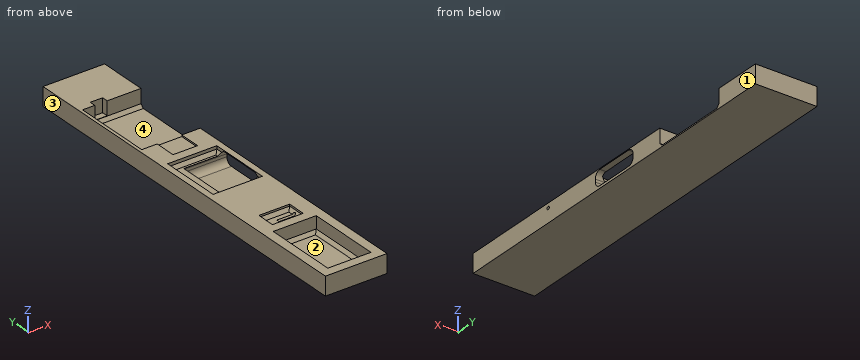
```python
from build123d import *

# Parameters (mm, degrees)
BOX038_W          = 4
BOX038_H          = 4
BOX038_DEPTH      = 10
BOX037_W          = 3
BOX037_H          = 6
BOX037_DEPTH      = 10
BOX036_W          = 2
BOX036_H          = 2.5
BOX036_DEPTH      = 10
BOX027_W          = 8.65
BOX027_H          = 8.3
BOX027_DEPTH      = 2.45
FILLET016_R       = 1
BOX034_W          = 7
BOX034_H          = 12
BOX034_DEPTH      = 3
CHAMFER002_SIZE   = 0.5
BOX033_W          = 8
BOX033_H          = 10
BOX033_DEPTH      = 10
CHAMFER001_SIZE   = 0.5
BOX032_W          = 5
BOX032_H          = 3
BOX032_DEPTH      = 10
CHAMFER_SIZE      = 0.5
BOX024_W          = 8.65
BOX024_H          = 8.3
BOX024_DEPTH      = 2.45
FILLET015_R       = 1
CYLINDER028_R     = 0.25
CYLINDER028_DEPTH = 10
BOX026_W          = 10
BOX026_H          = 13
BOX026_DEPTH      = 3
BOX014_W          = 10
BOX014_H          = 62
BOX014_DEPTH      = 3
CHAMFER003_SIZE   = 0.5


with BuildPart() as cubo032:
    # Box038 → Box038 (new body)
    with BuildSketch(Plane(origin=(127.5, 40, 4.75), x_dir=(1, 0, 0), z_dir=(0, 0, 1))):
        with Locations((2, 2)):
            Rectangle(BOX038_W, BOX038_H)
    extrude(amount=BOX038_DEPTH)


with BuildPart() as cubo031:
    # Box037 → Box037 (new body)
    with BuildSketch(Plane(origin=(128, 41, 4.75), x_dir=(1, 0, 0), z_dir=(0, 0, 1))):
        with Locations((1.5, 3)):
            Rectangle(BOX037_W, BOX037_H)
    extrude(amount=BOX037_DEPTH)


with BuildPart() as cubo030:
    # Box036 → Box036 (new body)
    with BuildSketch(Plane(origin=(127, 55, 2.75), x_dir=(1, 0, 0), z_dir=(0, 0, 1))):
        with Locations((1, 1.25)):
            Rectangle(BOX036_W, BOX036_H)
    extrude(amount=BOX036_DEPTH)


with BuildPart() as usb_c002:
    # Box027 → Box027 (new body)
    with BuildSketch(Plane.XY):
        with Locations((4.325, 4.15)):
            Rectangle(BOX027_W, BOX027_H)
    extrude(amount=BOX027_DEPTH)

    # Fillet016
    fillet016_edges = [usb_c002.edges().sort_by_distance(p)[0] for p in [
        (4.325, 0, 0),
        (4.325, 0, 2.45),
        (4.325, 8.3, 0),
        (4.325, 8.3, 2.45),
    ]]
    fillet(fillet016_edges, radius=FILLET016_R)


with BuildPart() as usb_c002_1:
    # Fillet016 placement: moved
    add(usb_c002.part.moved(Location((127.5, 29.35, 2.4))))


with BuildPart() as chamfer002:
    # Box034 → Box034 (new body)
    with BuildSketch(Plane(origin=(126, 4, 2.5), x_dir=(1, 0, 0), z_dir=(0, 0, 1))):
        with Locations((3.5, 6)):
            Rectangle(BOX034_W, BOX034_H)
    extrude(amount=BOX034_DEPTH)

    # Chamfer002
    chamfer002_edges = [chamfer002.edges().sort_by_distance(p)[0] for p in [
        (126, 10, 2.5),
        (133, 10, 2.5),
        (129.5, 4, 2.5),
        (129.5, 16, 2.5),
    ]]
    chamfer(chamfer002_edges, length=CHAMFER002_SIZE)


with BuildPart() as chamfer001:
    # Box033 → Box033 (new body)
    with BuildSketch(Plane(origin=(124, 28.5, 0), x_dir=(1, 0, 0), z_dir=(0, 0, 1))):
        with Locations((4, 5)):
            Rectangle(BOX033_W, BOX033_H)
    extrude(amount=BOX033_DEPTH)

    # Chamfer001
    chamfer001_edges = [chamfer001.edges().sort_by_distance(p)[0] for p in [
        (124, 33.5, 0),
        (132, 33.5, 0),
        (128, 28.5, 0),
        (128, 38.5, 0),
    ]]
    chamfer(chamfer001_edges, length=CHAMFER001_SIZE)


with BuildPart() as chamfer001_1:
    # Chamfer001 placement: moved
    add(chamfer001.part.moved(Location((1.5, 0, 4))))


with BuildPart() as chamfer_body:
    # Box032 → Box032 (new body)
    with BuildSketch(Plane(origin=(124, 14, 0), x_dir=(1, 0, 0), z_dir=(0, 0, 1))):
        with Locations((2.5, 1.5)):
            Rectangle(BOX032_W, BOX032_H)
    extrude(amount=BOX032_DEPTH)

    # Chamfer
    chamfer_edges = [chamfer_body.edges().sort_by_distance(p)[0] for p in [
        (124, 15.5, 0),
        (129, 15.5, 0),
        (126.5, 14, 0),
        (126.5, 17, 0),
    ]]
    chamfer(chamfer_edges, length=CHAMFER_SIZE)


with BuildPart() as chamfer_body_1:
    # Chamfer placement: moved
    add(chamfer_body.part.moved(Location((3, 3.5, 4.2))))


with BuildPart() as usb_c001:
    # Box024 → Box024 (new body)
    with BuildSketch(Plane.XY):
        with Locations((4.325, 4.15)):
            Rectangle(BOX024_W, BOX024_H)
    extrude(amount=BOX024_DEPTH)

    # Fillet015
    fillet015_edges = [usb_c001.edges().sort_by_distance(p)[0] for p in [
        (4.325, 0, 0),
        (4.325, 0, 2.45),
        (4.325, 8.3, 0),
        (4.325, 8.3, 2.45),
    ]]
    fillet(fillet015_edges, radius=FILLET015_R)


with BuildPart() as usb_c001_1:
    # Fillet015 placement: moved
    add(usb_c001.part.moved(Location((130, 29.35, 2.4))))


with BuildPart() as cilindro026:
    # Cylinder028 → Cylinder028 (new body)
    with BuildSketch(Plane(origin=(129, 19, 4.25), x_dir=(0, 1, 0), z_dir=(1, 0, 0))):
        Circle(CYLINDER028_R)
    extrude(amount=CYLINDER028_DEPTH)


with BuildPart() as obj1:
    # Box026 → Box026 (new body)
    with BuildSketch(Plane(origin=(125, 43.5, 2.2), x_dir=(1, 0, 0), z_dir=(0, 0, 1))):
        with Locations((5, 6.5)):
            Rectangle(BOX026_W, BOX026_H)
    extrude(amount=BOX026_DEPTH)


with BuildPart() as cut044:
    # Box014 → Box014 (new body)
    with BuildSketch(Plane(origin=(124.5, 2.5, 2), x_dir=(1, 0, 0), z_dir=(0, 0, 1))):
        with Locations((5, 31)):
            Rectangle(BOX014_W, BOX014_H)
    extrude(amount=BOX014_DEPTH)

    # Cut030: cut obj1
    add(obj1.part, mode=Mode.SUBTRACT)

    # Cut032: cut Cilindro026
    add(cilindro026.part, mode=Mode.SUBTRACT)

    # Cut033: cut USB-C001
    add(usb_c001_1.part, mode=Mode.SUBTRACT)

    # Cut038: cut Chamfer body
    add(chamfer_body_1.part, mode=Mode.SUBTRACT)

    # Cut039: cut Chamfer001
    add(chamfer001_1.part, mode=Mode.SUBTRACT)

    # Cut040: cut Chamfer002
    add(chamfer002.part, mode=Mode.SUBTRACT)

    # Cut041: cut USB-C002
    add(usb_c002_1.part, mode=Mode.SUBTRACT)

    # Chamfer003
    chamfer003_edges = [cut044.edges().sort_by_distance(p)[0] for p in [
        (129.75, 56.5, 2.2),
        (125, 50, 2.2),
        (129.75, 43.5, 2.2),
    ]]
    chamfer(chamfer003_edges, length=CHAMFER003_SIZE)

    # Cut042: cut Cubo030
    add(cubo030.part, mode=Mode.SUBTRACT)

    # Cut043: cut Cubo031
    add(cubo031.part, mode=Mode.SUBTRACT)

    # Cut044: cut Cubo032
    add(cubo032.part, mode=Mode.SUBTRACT)


solid = cut044.part
```
Read the model definition and answer for the solid it produces. Units are mm, in the model's axes. Face numbers are marked on the shaded views. Coordinates: 2 decimals unless noted, no trailing zeros. Order: outer loops, then holes, each group sorted by start corner. A loop starts at its lowest first (then second) coordinate and runs counter-clockwise, first axis right, second up. Notation, with made-up numbers: (35.5, 14.5) - (39.5, 14.5) arc R25 cw to (39.5, 36.5) - close; hole circle Ø10 at (-6.5, 14). An arc over 180 degrees is marked (long way). Answer as a JSON object with one key per item and string values. Group by question number.
Item 1: Section C-C (y = 7.5) is taken. Give the vertices of the cut face in (x, z).
Item 2: The mould has two halves that part along X. Classify the marked faces 1, 2, 3 and 4: +X half, -X half, draft (parallel to the pull), parting line (faces both ways), or undercut.
Item 3: Section A-A (y = 31.5) is taken. Give the vertices of the cut face in (x, z), plus the area to 3 significant figures.
Item 4: Flat-ended cylindrical pins translate along their axes: P1, Ø0.8, axis at x = 128, y = 57, coming from the +Z side; P2, Ø1.6, axis at x = 130, y = 19.5, coming from the +Z side. Find the tip coordinate at first contact, or state that the pin passes through.
Item 5: Section B-B (y = 48) is taken. Give the vertices of the cut face in (x, z).
Item 6: Consider probe 1 along Y at (x, z) = (129.5, 3.5); probe 2 along Y at (x, z) = (125.75, 4.8). Determine where each line is inside the solid, lowest interval first. Write a range as from..to.
Results are:
{
 "1": {"outline": "(124.5, 2) - (134.5, 2) - (134.5, 5) - (133, 5) - (133, 3) - (132.5, 2.5) - (126.5, 2.5) - (126, 3) - (126, 5) - (124.5, 5) - close"},
 "2": {"face 1": "+X half", "face 2": "undercut", "face 3": "-X half", "face 4": "draft"},
 "3": {"outline": "(124.5, 2) - (134.5, 2) - (134.5, 2.4) - (127.5, 2.4) - (127.5, 4) - (126, 4) - (125.5, 4.5) - (125.5, 5) - (124.5, 5) - close; (133.5, 4.85) - (134.5, 4.85) - (134.5, 5) - (133.5, 5) - close", "area": "10.1 mm^2"},
 "4": {"P1": "stops at z = 2.75", "P2": "stops at z = 4.5"},
 "5": {"outline": "(124.5, 2) - (134.5, 2) - (134.5, 2.2) - (125.5, 2.2) - (125, 2.7) - (125, 5) - (124.5, 5) - close"},
 "6": {"probe 1": "y = 2.5..4, 16..29.35, 37.65..43.5, 56.5..64.5", "probe 2": "y = 2.5..28.5, 38.5..43.5, 56.5..64.5"}
}
